```python
from build123d import *

# Parameters (mm, degrees)
BOSS_EXTRUDE1_DEPTH = 80
SKETCH3_W           = 40
SKETCH3_H           = 20
CUT_EXTRUDE1_DEPTH  = 139.564064606
FILLET1_R           = 5
CHAMFER1_SIZE       = 5
SKETCH4_R           = 10
CUT_EXTRUDE2_DEPTH  = 121
CHAMFER2_SIZE       = 5
FILLET2_R           = 5
CHAMFER3_SIZE       = 5
CHAMFER4_SIZE       = 5
CHAMFER5_SIZE       = 5
CHAMFER6_SIZE       = 5


with BuildPart() as part:
    # Sketch1 → Boss-Extrude1 (new body)
    with BuildSketch(Plane.XY):
        Polygon((0, 0), (-80, 0), (-80, 40), (-40, 40), (-40, 80), (0, 80), align=None)
    extrude(amount=BOSS_EXTRUDE1_DEPTH)

    # Sketch3 → Cut-Extrude1 (cut, through all)
    with BuildSketch(Plane(origin=(0, 0, 0), x_dir=(0, 0, -1), z_dir=(1, 0, 0))):
        with Locations((-40, 70)):
            Rectangle(SKETCH3_W, SKETCH3_H)
    extrude(amount=-CUT_EXTRUDE1_DEPTH, mode=Mode.SUBTRACT)

    # Fillet1
    fillet1_edges = [part.edges().sort_by_distance(p)[0] for p in [
        (-20, 80, 80),
        (-20, 80, 0),
    ]]
    fillet(fillet1_edges, radius=FILLET1_R)

    # Chamfer1
    chamfer1_edges = [part.edges().sort_by_distance(p)[0] for p in [
        (-20, 80, 60),
        (-20, 80, 20),
    ]]
    chamfer(chamfer1_edges, length=CHAMFER1_SIZE)

    # Sketch4 → Cut-Extrude2 (cut, through all)
    with BuildSketch(Plane(origin=(0, 40, 0), x_dir=(1, 0, 0), z_dir=(0, 1, 0))):
        with Locations(Location((-60, -40, 0), (0, 0, 270))):
            Circle(SKETCH4_R)
    extrude(amount=-CUT_EXTRUDE2_DEPTH, mode=Mode.SUBTRACT)

    # Chamfer2
    chamfer2_edges = [part.edges().sort_by_distance(p)[0] for p in [
        (-80, 40, 40),
    ]]
    chamfer(chamfer2_edges, length=CHAMFER2_SIZE)

    # Fillet2
    fillet2_edges = [part.edges().sort_by_distance(p)[0] for p in [
        (-40, 40, 40),
    ]]
    fillet(fillet2_edges, radius=FILLET2_R)

    # Chamfer3
    chamfer3_edges = [part.edges().sort_by_distance(p)[0] for p in [
        (-80, 0, 40),
    ]]
    chamfer(chamfer3_edges, length=CHAMFER3_SIZE)

    # Chamfer4
    chamfer4_edges = [part.edges().sort_by_distance(p)[0] for p in [
        (0, 0, 40),
    ]]
    chamfer(chamfer4_edges, length=CHAMFER4_SIZE)

    # Chamfer5
    chamfer5_edges = [part.edges().sort_by_distance(p)[0] for p in [
        (0, 60, 40),
    ]]
    chamfer(chamfer5_edges, length=CHAMFER5_SIZE)

    # Chamfer6
    chamfer6_edges = [part.edges().sort_by_distance(p)[0] for p in [
        (-40, 60, 40),
    ]]
    chamfer(chamfer6_edges, length=CHAMFER6_SIZE)


solid = part.part
```
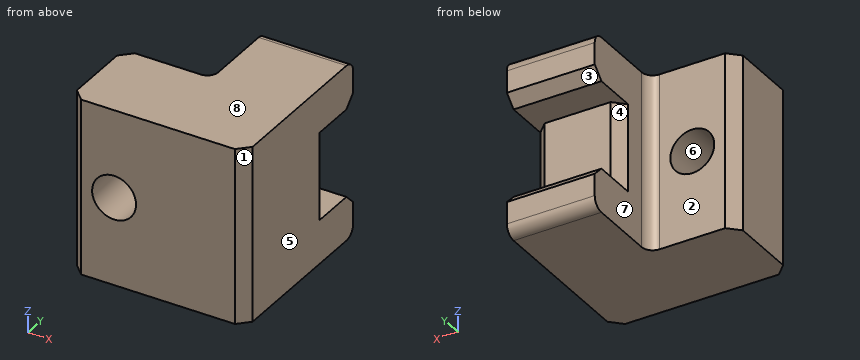
Can you work these out from the model? Positions are in its coordinate system, mm. Face numbers are marked on the shaded views. A direction names the side the tool comes from. Give positions to 0.01 mm unless a question says otherwise; leave off trailing zeros. Order: outer loops, then holes, each group sorted by start corner. A loop starts at its lowest first (then second) coordinate and runs counter-clockwise, first axis right, second up. Notation, with made-up numbers: (75.25, -15) - (92.25, -15) arc R21 ccw to (92.25, -8) - close; hole circle Ø8 at (35, 46.25). An arc over 180 degrees is marked (long way). Use a Markdown table: item, result. Add a question column.
Q1. I'm going to push flat-ended pins straight in: pin 1 (1.5 mm diameter, centred on x = -66, z = 58, fed in from +Y); pin 2 (10.5 mm diameter, centred on y = 63.5, z = 41, fed in from -X); pin 3 (3 mm diameter, centred on y = 40.5, z = 21, fed in from -X). Where does each tip first touch, or does it pass through?
Q2. If we section it at A-A on x = -60: Write out the boundary of the cut face in (y, z).
Q3. If we mould it in two halves opening along X, with no side actions, what happens to the marked faces 6, 7 and 8? For each: released by +X, released by -X, zero draft, split by the parting line, or undercut.
Q4. On a 3-axis mill with a long thin cutter (end or side, diameter ignored), from which of +Z, -Z, +X, -X, +Y, -Y can I reach the whole of each face in a straight line? I mean the marked faces 1, 2, 3, 4 and 5. Say none if no direction works.
Q5. If we section it at C-C on z = 70.5: Write out the boundary of the cut face in (x, y), plus the area to 3 significant figures.
Q6. If we section it at D-D on y = 29.5: Write out the boundary of the cut face in (x, z), plus the area to 3 significant figures.
Q7. If we section it at B-B on z = 40: Write out the boundary of the cut face in (x, y), plus the area to 3 significant figures.
Q8. Please list where these lines run through material, in increasing order: line 1 along X through (y, z) = (28, 40); line 2 along Z through (x, y) = (-4.5, 74.5); line 3 along Y through (x, z) = (-45.5, 21.5).
Answers follow:
| question | item | result |
|---|---|---|
| 1 | pin 1 | stops at y = 40 |
| 1 | pin 2 | stops at x = -36.75 |
| 1 | pin 3 | stops at x = -76 |
| 2 | outline | (0, 0) - (40, 0) - (40, 30) - (0, 30) - close; (0, 50) - (40, 50) - (40, 80) - (0, 80) - close |
| 3 | face 6 | undercut |
| 3 | face 7 | released by -X |
| 3 | face 8 | zero draft |
| 4 | face 1 | +Z, -Z, +X, -Y |
| 4 | face 2 | +Z, -Z, -X, +Y |
| 4 | face 3 | +X, -X, +Y |
| 4 | face 4 | -X, +Y |
| 4 | face 5 | +Z, -Z, +X, +Y, -Y |
| 5 | outline | (-80, 5) - (-75, 0) - (-5, 0) - (0, 5) - (0, 80) - (-40, 80) - (-40, 45) arc R5 cw to (-45, 40) - (-75, 40) - (-80, 35) - close |
| 5 | area | 4,770 mm^2 |
| 6 | outline | (-80, 0) - (0, 0) - (0, 80) - (-80, 80) - close; hole circle Ø20 at (-60, 40) |
| 6 | area | 6,090 mm^2 |
| 7 | outline | (-80, 5) - (-75, 0) - (-70, 0) - (-70, 40) - (-75, 40) - (-80, 35) - close; (-50, 0) - (-5, 0) - (0, 5) - (0, 55) - (-5, 60) - (-35, 60) - (-40, 55) - (-40, 45) arc R5 cw to (-45, 40) - (-50, 40) - close |
| 7 | area | 3,140 mm^2 |
| 8 | line 1 | x = -80 to -70, -50 to 0 |
| 8 | line 2 | z = 0 to 20, 60 to 80 |
| 8 | line 3 | y = 0 to 40 |
